```python
from build123d import *
from build123d.topology import SkipClean

# Parameters (mm, degrees)
SKETCH_1_R      = 2
SKETCH_1_R_2    = 1.25
EXTRUDE_1_DEPTH = 3
SKETCH_2_R      = 2
SKETCH_2_R_2    = 1.25
EXTRUDE_2_DEPTH = 3
SKETCH_3_R      = 1.5
EXTRUDE_3_DEPTH = 3
EXTRUDE_4_DEPTH = 3


with BuildPart() as part:
    # 草图1 → 凸台-拉伸1 (new body)
    # profile 1 of 12: a face of its own
    with BuildSketch(Plane(origin=(0, 0, 0), x_dir=(1, 0, 0), z_dir=(0, 1, 0))):
        with BuildLine():
            ThreePointArc((-27, -24.5), (-27.585786438, -25.914213562), (-29, -26.5))
            Line((-29, -26.5), (29, -26.5))
            ThreePointArc((29, -26.5), (27.585786438, -25.914213562), (27, -24.5))
            Line((27, -24.5), (27, -22.5))
            Line((27, -22.5), (-27, -22.5))
            Line((-27, -22.5), (-27, -24.5))
        make_face()
    # profile 2 of 12: a face of its own
    with BuildSketch(Plane(origin=(0, 0, 0), x_dir=(1, 0, 0), z_dir=(0, 1, 0))):
        with BuildLine():
            Line((29, -22.5), (27, -22.5))
            Line((27, -22.5), (27, -24.5))
            ThreePointArc((27, -24.5), (27.585786438, -23.085786438), (29, -22.5))
        make_face()
    # profile 3 of 12: a face of its own
    with BuildSketch(Plane(origin=(0, 0, 0), x_dir=(1, 0, 0), z_dir=(0, 1, 0))):
        with Locations((29, -24.5)):
            Circle(SKETCH_1_R)
        with Locations(Location((29, -24.5, 0), (0, 0, 270))):
            Circle(SKETCH_1_R_2, mode=Mode.SUBTRACT)
    # profile 4 of 12: a face of its own
    with BuildSketch(Plane(origin=(0, 0, 0), x_dir=(1, 0, 0), z_dir=(0, 1, 0))):
        with BuildLine():
            Line((31, -24.5), (31, 24.5))
            ThreePointArc((31, 24.5), (30.414213562, 23.085786438), (29, 22.5))
            Line((29, 22.5), (27, 22.5))
            Line((27, 22.5), (27, -22.5))
            Line((27, -22.5), (29, -22.5))
            ThreePointArc((29, -22.5), (30.414213562, -23.085786438), (31, -24.5))
        make_face()
    # profile 5 of 12: a face of its own
    with BuildSketch(Plane(origin=(0, 0, 0), x_dir=(1, 0, 0), z_dir=(0, 1, 0))):
        with BuildLine():
            ThreePointArc((-29, 22.5), (-30.414213562, 23.085786438), (-31, 24.5))
            Line((-31, 24.5), (-31, -24.5))
            ThreePointArc((-31, -24.5), (-30.414213562, -23.085786438), (-29, -22.5))
            Line((-29, -22.5), (-27, -22.5))
            Line((-27, -22.5), (-27, 22.5))
            Line((-27, 22.5), (-29, 22.5))
        make_face()
    # profile 6 of 12: a face of its own
    with BuildSketch(Plane(origin=(0, 0, 0), x_dir=(1, 0, 0), z_dir=(0, 1, 0))):
        with Locations((-29, -24.5)):
            Circle(SKETCH_1_R)
        with Locations(Location((-29, -24.5, 0), (0, 0, 270))):
            Circle(SKETCH_1_R_2, mode=Mode.SUBTRACT)
    # profile 7 of 12: a face of its own
    with BuildSketch(Plane(origin=(0, 0, 0), x_dir=(1, 0, 0), z_dir=(0, 1, 0))):
        with BuildLine():
            Line((-27, -22.5), (-29, -22.5))
            ThreePointArc((-29, -22.5), (-27.585786438, -23.085786438), (-27, -24.5))
            Line((-27, -24.5), (-27, -22.5))
        make_face()
    # profile 8 of 12: a face of its own
    with BuildSketch(Plane(origin=(0, 0, 0), x_dir=(1, 0, 0), z_dir=(0, 1, 0))):
        with BuildLine():
            ThreePointArc((29, 22.5), (27.585786438, 23.085786438), (27, 24.5))
            Line((27, 24.5), (27, 22.5))
            Line((27, 22.5), (29, 22.5))
        make_face()
    # profile 9 of 12: a face of its own
    with BuildSketch(Plane(origin=(0, 0, 0), x_dir=(1, 0, 0), z_dir=(0, 1, 0))):
        with Locations((29, 24.5)):
            Circle(SKETCH_1_R)
        with Locations(Location((29, 24.5, 0), (0, 0, 270))):
            Circle(SKETCH_1_R_2, mode=Mode.SUBTRACT)
    # profile 10 of 12: a face of its own
    with BuildSketch(Plane(origin=(0, 0, 0), x_dir=(1, 0, 0), z_dir=(0, 1, 0))):
        with BuildLine():
            Line((29, 26.5), (-29, 26.5))
            ThreePointArc((-29, 26.5), (-27.585786438, 25.914213562), (-27, 24.5))
            Line((-27, 24.5), (-27, 22.5))
            Line((-27, 22.5), (27, 22.5))
            Line((27, 22.5), (27, 24.5))
            ThreePointArc((27, 24.5), (27.585786438, 25.914213562), (29, 26.5))
        make_face()
    # profile 11 of 12: a face of its own
    with BuildSketch(Plane(origin=(0, 0, 0), x_dir=(1, 0, 0), z_dir=(0, 1, 0))):
        with BuildLine():
            ThreePointArc((-27, 24.5), (-27.585786438, 23.085786438), (-29, 22.5))
            Line((-29, 22.5), (-27, 22.5))
            Line((-27, 22.5), (-27, 24.5))
        make_face()
    # profile 12 of 12: a face of its own
    with BuildSketch(Plane(origin=(0, 0, 0), x_dir=(1, 0, 0), z_dir=(0, 1, 0))):
        with Locations((-29, 24.5)):
            Circle(SKETCH_1_R)
        with Locations(Location((-29, 24.5, 0), (0, 0, 270))):
            Circle(SKETCH_1_R_2, mode=Mode.SUBTRACT)
    extrude(amount=EXTRUDE_1_DEPTH)

    # 草图2 → 凸台-拉伸2 (add)
    # profile 1 of 4: a face of its own
    with SkipClean():  # the faces are left unmerged after this step: merging them gives an invalid solid
        with BuildSketch(Plane(origin=(0, 3, 0), x_dir=(1, 0, 0), z_dir=(0, 1, 0))):
            with Locations(Location((-29, 24.5, 0), (0, 0, 90))):
                Circle(SKETCH_2_R)
            with Locations(Location((-29, 24.5, 0), (0, 0, 270))):
                Circle(SKETCH_2_R_2, mode=Mode.SUBTRACT)
        # profile 2 of 4: a face of its own
        with BuildSketch(Plane(origin=(0, 3, 0), x_dir=(1, 0, 0), z_dir=(0, 1, 0))):
            with Locations(Location((29, 24.5, 0), (0, 0, 90))):
                Circle(SKETCH_2_R)
            with Locations(Location((29, 24.5, 0), (0, 0, 270))):
                Circle(SKETCH_2_R_2, mode=Mode.SUBTRACT)
        # profile 3 of 4: a face of its own
        with BuildSketch(Plane(origin=(0, 3, 0), x_dir=(1, 0, 0), z_dir=(0, 1, 0))):
            with Locations(Location((-29, -24.5, 0), (0, 0, 270))):
                Circle(SKETCH_2_R)
            with Locations(Location((-29, -24.5, 0), (0, 0, 270))):
                Circle(SKETCH_2_R_2, mode=Mode.SUBTRACT)
        # profile 4 of 4: a face of its own
        with BuildSketch(Plane(origin=(0, 3, 0), x_dir=(1, 0, 0), z_dir=(0, 1, 0))):
            with Locations(Location((29, -24.5, 0), (0, 0, 270))):
                Circle(SKETCH_2_R)
            with Locations(Location((29, -24.5, 0), (0, 0, 270))):
                Circle(SKETCH_2_R_2, mode=Mode.SUBTRACT)
        extrude(amount=EXTRUDE_2_DEPTH)

    # 草图3 → 凸台-拉伸3 (add)
    # profile 1 of 4: a face of its own
    with BuildSketch(Plane.XZ):
        with BuildLine():
            Line((-31, 24.5), (-31, 31.727166486))
            Line((-31, 31.727166486), (-27, 31.727166486))
            Line((-27, 31.727166486), (-27, 26.5))
            Line((-27, 26.5), (-29, 26.5))
            ThreePointArc((-29, 26.5), (-30.414213562, 25.914213562), (-31, 24.5))
        make_face()
        with Locations(Location((-29, 29.5, 0), (0, 0, 270))):
            Circle(SKETCH_3_R, mode=Mode.SUBTRACT)
    # profile 2 of 4: a face of its own
    with BuildSketch(Plane.XZ):
        with BuildLine():
            Line((29, 26.5), (27, 26.5))
            Line((27, 26.5), (27, 31.727166486))
            Line((27, 31.727166486), (31, 31.727166486))
            Line((31, 31.727166486), (31, 24.5))
            ThreePointArc((31, 24.5), (30.414213562, 25.914213562), (29, 26.5))
        make_face()
        with Locations(Location((29, 29.5, 0), (0, 0, 90))):
            Circle(SKETCH_3_R, mode=Mode.SUBTRACT)
    # profile 3 of 4: a face of its own
    with BuildSketch(Plane.XZ):
        with BuildLine():
            Line((31, -24.5), (31, -31.727166486))
            Line((31, -31.727166486), (27, -31.727166486))
            Line((27, -31.727166486), (27, -26.5))
            Line((27, -26.5), (29, -26.5))
            ThreePointArc((29, -26.5), (30.414213562, -25.914213562), (31, -24.5))
        make_face()
        with Locations(Location((29, -29.5, 0), (0, 0, 270))):
            Circle(SKETCH_3_R, mode=Mode.SUBTRACT)
    # profile 4 of 4: a face of its own
    with BuildSketch(Plane.XZ):
        with BuildLine():
            Line((-29, -26.5), (-27, -26.5))
            Line((-27, -26.5), (-27, -31.727166486))
            Line((-27, -31.727166486), (-31, -31.727166486))
            Line((-31, -31.727166486), (-31, -24.5))
            ThreePointArc((-31, -24.5), (-30.414213562, -25.914213562), (-29, -26.5))
        make_face()
        with Locations(Location((-29, -29.5, 0), (0, 0, 90))):
            Circle(SKETCH_3_R, mode=Mode.SUBTRACT)
    extrude(amount=-EXTRUDE_3_DEPTH)

    # 草图4 → 凸台-拉伸4 (add)
    with BuildSketch(Plane.XZ):
        Polygon((-31, 26.5), (-33, 26.5), (-33, 31.727166486), (-33, 33.727166486), (-25, 33.727166486), (-25, 26.5), (-27, 26.5), (-27, 31.727166486), (-31, 31.727166486), align=None)
        Polygon((27, 31.727166486), (27, 26.5), (25, 26.5), (25, 33.727166486), (33, 33.727166486), (33, 31.727166486), (33, 26.5), (31, 26.5), (31, 31.727166486), align=None)
        Polygon((31, -26.5), (33, -26.5), (33, -31.727166486), (33, -33.727166486), (25, -33.727166486), (25, -26.5), (27, -26.5), (27, -31.727166486), (31, -31.727166486), align=None)
        Polygon((-27, -31.727166486), (-27, -26.5), (-25, -26.5), (-25, -33.727166486), (-33, -33.727166486), (-33, -31.727166486), (-33, -26.5), (-31, -26.5), (-31, -31.727166486), align=None)
    extrude(amount=-EXTRUDE_4_DEPTH)


solid = part.part
```
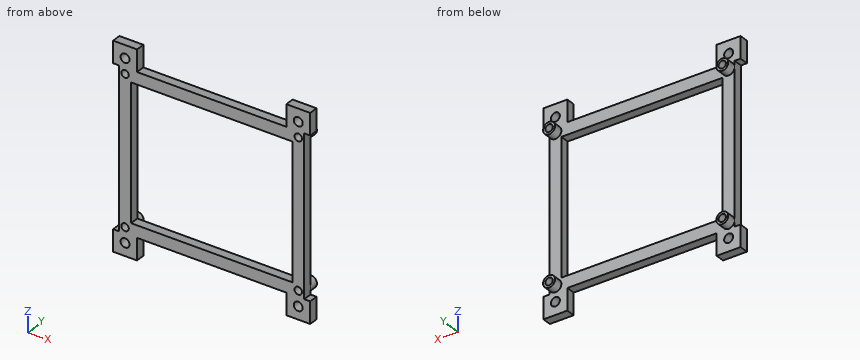
Geometry check sheet. Reference: the model listing, model coordinates, mm. Coordinates: 2 decimals unless noted, no trailing zeros. Order: outer loops, then holes, each group sorted by start corner. A loop starts at its lowest first (then second) coordinate and runs counter-clockwise, first axis right, second up.
Item 1: Scan lines: line 1 along X through (y, z) = (4.6, 24.5); line 2 along X through (y, z) = (1.8, -24.5); line 3 along X through (y, z) = (1.9, -29.5). Record each from-to range of solid material in increasing order.
Item 2: Section check A-A (y = 3.8). Enter the section's corners in (x, z), plus the area to 3 significant figures.
Item 3: Depth check by flat-ended pin: pin 1 (1.5 mm diameter, centred on x = -9, y = 2, fed in from -Z); pin 2 (1.5 mm diameter, centred on x = 3, y = 1, fed in from +Z); pin 3 (1.5 mm diameter, centred on y = 1.5, z = -3, fed in from -X). Enter the tip coordinate at first touch or a pass-through.
Item 4: Section check B-B (z = -29.5). Enter the section's corners in (x, y).
Item 5: Section check D-D (z = -9). Enter the section's corners in (x, y), plus the area to 3 significant figures.
Item 6: Section check C-C (x = -2). Enter the section's corners in (y, z).
Check sheet entries:
1. line 1: x = -31 to -30.25, -27.75 to -27, 27 to 27.75, 30.25 to 31
1. line 2: x = -31 to -30.25, -27.75 to 27.75, 30.25 to 31
1. line 3: x = -33 to -30.5, -27.5 to -25, 25 to 27.5, 30.5 to 33
2. outline: circle Ø4 at (-29, -24.5); circle Ø4 at (-29, 24.5); circle Ø4 at (29, -24.5); circle Ø4 at (29, 24.5); hole circle Ø2.5 at (-29, -24.5); hole circle Ø2.5 at (-29, 24.5); hole circle Ø2.5 at (29, -24.5); hole circle Ø2.5 at (29, 24.5)
2. area: 30.6 mm2
3. pin 1: stops at z = -26.5
3. pin 2: stops at z = 26.5
3. pin 3: stops at x = -31
4. outline: (-33, 0) - (-30.5, 0) - (-30.5, 3) - (-33, 3) - close; (-27.5, 0) - (-25, 0) - (-25, 3) - (-27.5, 3) - close; (25, 0) - (27.5, 0) - (27.5, 3) - (25, 3) - close; (30.5, 0) - (33, 0) - (33, 3) - (30.5, 3) - close
5. outline: (-31, 0) - (-27, 0) - (-27, 3) - (-31, 3) - close; (27, 0) - (31, 0) - (31, 3) - (27, 3) - close
5. area: 24.0 mm2
6. outline: (0, -26.5) - (3, -26.5) - (3, -22.5) - (0, -22.5) - close; (0, 22.5) - (3, 22.5) - (3, 26.5) - (0, 26.5) - close
